Part model, mm, in its own coordinate system. Face numbers are marked on the shaded views. Coordinates: 2 decimals unless noted, no trailing zeros. Write item = value, one per line.
from build123d import *

# Parameters (mm, degrees)
F1_DEPTH  = 201
F4_DEPTH  = 30
F7_DEPTH  = 388.393305
F9_DEPTH  = 20
F11_DEPTH = 20
F13_DEPTH = 60.536898
F15_DEPTH = 60.536898
F17_DEPTH = 140.001
F19_DEPTH = 456.084874
F21_DEPTH = 456.084874


with BuildPart() as f1:
    # F0 (on Front) → F1 (new body)
    with BuildSketch(Plane.XZ):
        Polygon((-83.5, 78), (0, 78), (83.5, 78), (93.892305, 60), (93.892305, 0), (95.892305, 0), (95.892305, 60.535898), (84.654701, 80), (0, 80), (-84.654701, 80), (-95.892305, 60.535898), (-95.892305, 0), (-93.892305, 0), (-93.892305, 60), align=None)
    extrude(amount=-F1_DEPTH)



with BuildPart() as f4:
    # F3 (on offset) → F4 (new body)
    with BuildSketch(Plane.XZ.offset(-412.5)):
        Polygon((212.5, 140), (0, 140), (-212.5, 140), (-292.5, 60), (-292.5, 0), (-290.5, 0), (-290.5, 59.171573), (-211.671573, 138), (0, 138), (211.671573, 138), (290.5, 59.171573), (290.5, 0), (292.5, 0), (292.5, 60), align=None)
    extrude(amount=-F4_DEPTH)


with BuildPart() as f1_1:
    add(f1.part)

    add(f4.part)  # F5 merges F4
    # F4_face (on face) → F5 section 0
    with BuildSketch(Plane(origin=(0, 412.5, 110.440506), x_dir=(1, 0, 0), z_dir=(0, -1, 0))):
        Polygon((211.671573, 27.559494), (290.5, -51.268933), (290.5, -110.440506), (292.5, -110.440506), (292.5, -50.440506), (212.5, 29.559494), (-212.5, 29.559494), (-292.5, -50.440506), (-292.5, -110.440506), (-290.5, -110.440506), (-290.5, -51.268933), (-211.671573, 27.559494), align=None)
    # F1_face (on face) → F5 section 1
    with BuildSketch(Plane(origin=(0, 201, 60.03778), x_dir=(1, 0, 0), z_dir=(0, 1, 0))):
        Polygon((-95.892305, 60.03778), (-95.892305, -0.498118), (-84.654701, -19.96222), (84.654701, -19.96222), (95.892305, -0.498118), (95.892305, 60.03778), (93.892305, 60.03778), (93.892305, 0.03778), (83.5, -17.96222), (-83.5, -17.96222), (-93.892305, 0.03778), (-93.892305, 60.03778), align=None)
    loft()

    # F6 (on face) → F7 (cut, through all)
    with BuildSketch(Plane(origin=(-95.892305, 0, 0), x_dir=(0, -1, 0), z_dir=(-1, 0, 0))):
        Polygon((-163, 23), (-201, 23), (-201, 0), (0, 0), (0, 60), (-38.000001, 59.923097), (-38.000001, 60.535898), (-98, 60.527767), align=None)
    extrude(amount=-F7_DEPTH, mode=Mode.SUBTRACT)

    # F8 (on face) → F9 (join)
    with BuildSketch(Plane(origin=(-95.892305, 0, 0), x_dir=(0, -1, 0), z_dir=(-1, 0, 0))):
        Polygon((0, 60.535898), (-38.000001, 60.535898), (-38.000001, 59.923097), (0, 60), align=None)
    extrude(amount=F9_DEPTH)

    # F10 (on face) → F11 (join)
    with BuildSketch(Plane.YZ.offset(95.892305)):
        Polygon((0, 60.535898), (0, 60), (38.000001, 59.923097), (38.000001, 60.535898), align=None)
    extrude(amount=F11_DEPTH)

    # F12 (on face) → F13 (cut, through all)
    with BuildSketch(Plane.XY.offset(60.535898)):
        with BuildLine():
            ThreePointArc((-102.392305, 30.5), (-105.892305, 34), (-109.392305, 30.5))
            Line((-109.392305, 30.5), (-109.392305, 7.5))
            ThreePointArc((-109.392305, 7.5), (-105.892305, 4), (-102.392305, 7.5))
            Line((-102.392305, 7.5), (-102.392305, 30.5))
        make_face()
    extrude(amount=-F13_DEPTH, mode=Mode.SUBTRACT)

    # F14 (on face) → F15 (cut, through all)
    with BuildSketch(Plane.XY.offset(60.535898)):
        with BuildLine():
            ThreePointArc((109.392305, 30.5), (105.892305, 34), (102.392305, 30.5))
            Line((102.392305, 30.5), (102.392305, 7.5))
            ThreePointArc((102.392305, 7.5), (105.892305, 4), (109.392305, 7.5))
            Line((109.392305, 7.5), (109.392305, 30.5))
        make_face()
    extrude(amount=-F15_DEPTH, mode=Mode.SUBTRACT)

    # F16 (on face) → F17 (cut, through all)
    with BuildSketch(Plane.XY.offset(140)):
        with BuildLine():
            Line((-76.5, 427), (-76.5, 433))
            ThreePointArc((-76.5, 433), (-80, 436.5), (-83.5, 433))
            Line((-83.5, 433), (-83.5, 427))
            ThreePointArc((-83.5, 427), (-80, 423.5), (-76.5, 427))
        make_face()
        with BuildLine():
            Line((83.5, 427), (83.5, 433))
            ThreePointArc((83.5, 433), (80, 436.5), (76.5, 433))
            Line((76.5, 433), (76.5, 427))
            ThreePointArc((76.5, 427), (80, 423.5), (83.5, 427))
        make_face()
    extrude(amount=-F17_DEPTH, mode=Mode.SUBTRACT)

    # F18 (on face) → F19 (cut, through all)
    with BuildSketch(Plane(origin=(-176.25, 0, 176.25), x_dir=(0.707107, 0, 0.707107), z_dir=(-0.707107, 0, 0.707107))):
        with BuildLine():
            Line((-102.265242, 436), (-120.265242, 436))
            ThreePointArc((-120.265242, 436), (-126.265242, 430), (-120.265242, 424))
            Line((-120.265242, 424), (-102.265242, 424))
            ThreePointArc((-102.265242, 424), (-96.265242, 430), (-102.265242, 436))
        make_face()
    extrude(amount=-F19_DEPTH, mode=Mode.SUBTRACT)

    # F20 (on face) → F21 (cut, through all)
    with BuildSketch(Plane(origin=(176.25, 0, 176.25), x_dir=(0.707107, 0, -0.707107), z_dir=(0.707107, 0, 0.707107))):
        with BuildLine():
            ThreePointArc((120.265242, 424), (126.265242, 430), (120.265242, 436))
            Line((120.265242, 436), (102.265242, 436))
            ThreePointArc((102.265242, 436), (96.265242, 430), (102.265242, 424))
            Line((102.265242, 424), (120.265242, 424))
        make_face()
    extrude(amount=-F21_DEPTH, mode=Mode.SUBTRACT)


solid = f1_1.part
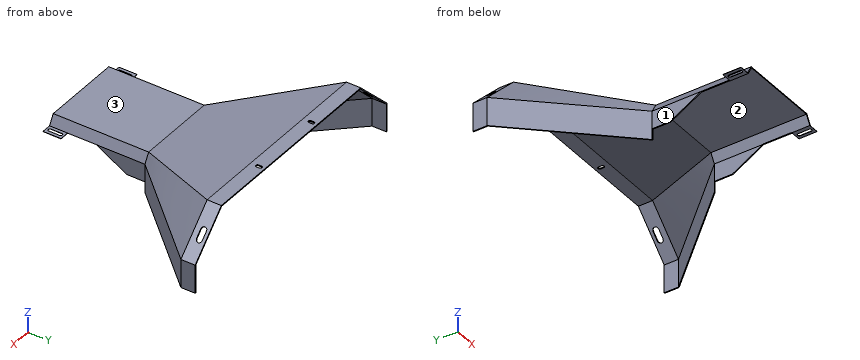
Q1. Mould opens along X. For the marked faces 1, 2 and 3 say: released by +X, released by -X, zero draft, split by the parting line, or undercut.
Model answer:
face_1 = released by -X
face_2 = undercut
face_3 = zero draft
Q2. Pin check, flat tips, straight feed: pin 1 (24 mm diameter, centred on x = 13, y = 430.5, fed in from -Z); pin 2 (0.5 mm diameter, centred on x = -102.5, z = 60, fed in from +Y); pin 3 (0.6 mm diameter, centred on y = 429.5, z = 139, fed in from -X). Stop position of each tip, or through.
Model answer:
pin_1 = 138
pin_2 = 210.61
pin_3 = -213.8
Q3. Probe line 1 (X direction, y = 402, z = 57.5); line 2 (X direction, y = 394, z = 35); line 3 (Z direction, x = 23.5, y = 424.5). List the from-to ranges inside material, lowest first. Write a range as from..to.
Model answer:
line_1 = -282.74..-280.74, 280.74..282.74
line_2 = -275.3..-273.3, 273.3..275.3
line_3 = 138..140
